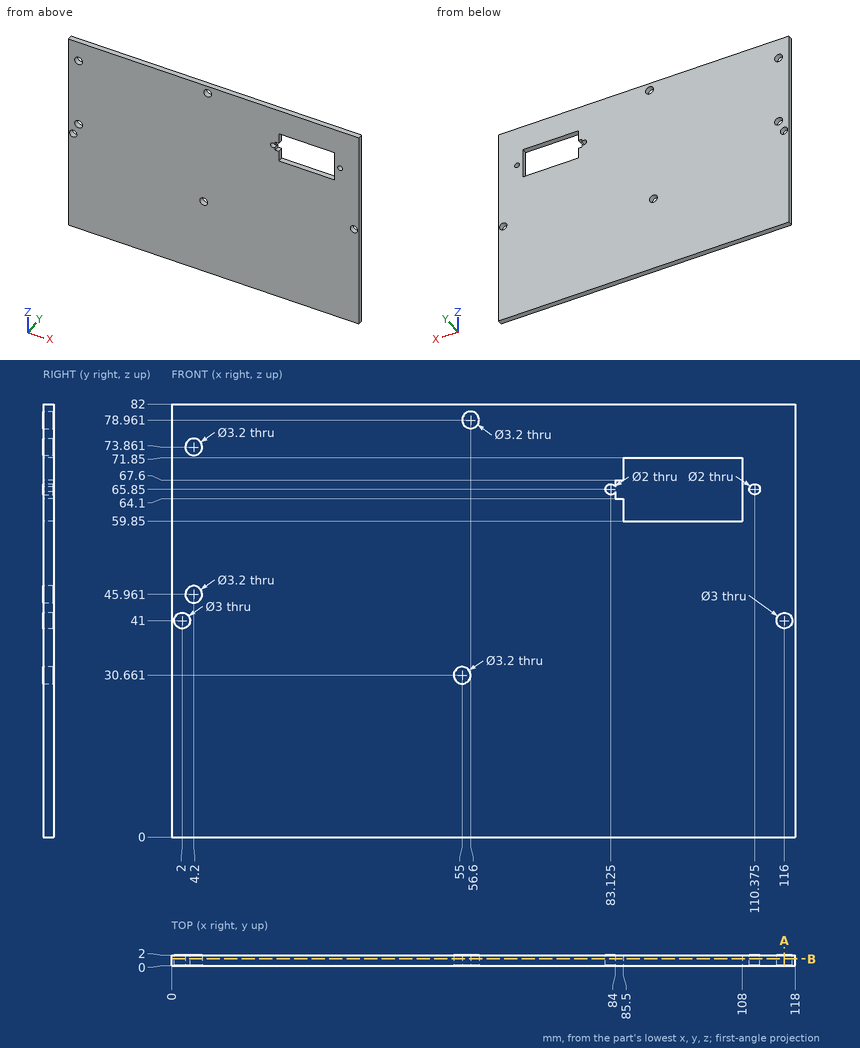
Job drawing, mm, ordinate dimensions from the low corner. One solid piece. Round coordinates to 2 decimals unless told otherwise and drop trailing zeros. Write each loop counter-clockwise with the first axis right and the second up, starting at its lowest first coordinate (ties: lowest second). Pieces come first, ordered by that corner, then holes. Notation, with made-up numbers: (-35, -21.5) -> (7, -21.5) arc R28 ccw to (7, 14.5) -> close; hole circle Ø4 at (-16.75, 63.25). An arc over 180 degrees is marked (long way). Answer as a JSON object with one key per item and string values.
(1) Probe probe 1 along X at (y, z) = (1.65, 41); probe 2 along X at (y, z) = (0.8, 65.85) (1 decimal); probe 3 along Z at (x, y) = (86.5, 1.7). List the from-to ranges inside material, lowest first. Write a range as [from, to].
Reported:
{"probe 1": "x = [0, 0.5], [3.5, 114.5], [117.5, 118]", "probe 2": "x = [0, 82.1], [108, 109.4], [111.4, 118]", "probe 3": "z = [0, 59.85], [71.85, 82]"}
(2) Band-saw the part on B-B, the plane y = 1.3. Count the separate pieces of the cut face and the enclosed holes in it, then the cut area to 3 significant figures.
Reported:
{"separate pieces": "1", "enclosed holes": "8", "area": "9,350 mm^2"}
(3) Band-saw the part on A-A, the plane x = 116. List the corners of the cut face in (y, z).
Reported:
{"outline": "(0, 0) -> (2, 0) -> (2, 39.5) -> (0, 39.5) -> close; (0, 42.5) -> (2, 42.5) -> (2, 82) -> (0, 82) -> close"}
